Part model, mm, in its own coordinate system. A direction names the side the tool comes from. Give positions to 0.01 mm unless a question says otherwise; leave off trailing zeros. Write each loop counter-clockwise with the first axis right and the second up, starting at its lowest first coordinate (ties: lowest second). Pieces come first, ordered by that corner, then holes. Notation, with made-up numbers: M 20.5,23.5 L 71.5,23.5 A20 cw 71.5,34.5 Z; hole C -31,2 d2. An arc over 180 degrees is marked long. Write item = value, one per line. Start each with the question number.
from build123d import *

# Parameters (mm, degrees)
SKETCH_2_R          = 3
SKETCH_2_R_2        = 0.75
CUT_EXTRUDE_1_DEPTH = 10
EXTRUDE_START       = -3.5
SKETCH_3_R          = 3
SKETCH_3_R_2        = 1.5
EXTRUDE_1_DEPTH     = 2.9


with BuildPart() as part:
    # 草图1 → 旋转1 (revolve)
    with BuildSketch(Plane.XY, mode=Mode.PRIVATE) as revolve_1_sk:
        Polygon((0, -0.6), (-3.55, -0.6), (-4.836704152, 0), (-10.35, 0), (-10.35, 2.6), (-4.3, 2.6), (-4.3, 5.8), (0, 5.8), align=None)
    revolve(revolve_1_sk.sketch.rotate(Axis((0, 0, 0), (0, 1, 0)), 270), axis=Axis((0, 0, 0), (0, 1, 0)))

    # 草图2 → 切除-拉伸1 (cut)
    with BuildSketch(Plane(origin=(0, 5.8, 0), x_dir=(1, 0, 0), z_dir=(0, 1, 0))):
        with Locations(Location((0, 0, 0), (0, 0, 270))):
            Circle(SKETCH_2_R)
        with Locations(Location((0, 7.25, 0), (0, 0, 270))):
            Circle(SKETCH_2_R_2)
        with Locations(Location((7.25, 0, 0), (0, 0, 270))):
            Circle(SKETCH_2_R_2)
        with Locations(Location((0, -7.25, 0), (0, 0, 270))):
            Circle(SKETCH_2_R_2)
        with Locations(Location((-7.25, 0, 0), (0, 0, 270))):
            Circle(SKETCH_2_R_2)
    extrude(amount=-CUT_EXTRUDE_1_DEPTH, mode=Mode.SUBTRACT)

    # 草图3 → 凸台-拉伸1 (add)
    with BuildSketch(Plane(origin=(0, 5.8, 0), x_dir=(1, 0, 0), z_dir=(0, 1, 0)).offset(EXTRUDE_START)):
        with Locations(Location((0, 0, 0), (0, 0, 270))):
            Circle(SKETCH_3_R)
        with Locations(Location((0, 0, 0), (0, 0, 270))):
            Circle(SKETCH_3_R_2, mode=Mode.SUBTRACT)
    extrude(amount=-EXTRUDE_1_DEPTH)


solid = part.part
Q1. Slice it at B-B (z = 0). Give the cut face in (x, y), and give its area (3 significant figures).
Q2. Slice it at C-C (y = 0.5). Give the cut face in (x, z), and give its area (3 significant figures).
Q3. Slice it at D-D (z = 7.25). Give the cut face in (x, y).
Q4. Drop flat-ended pins along their axis: P1, Ø3, axis at x = 4, y = 3.5, coming from the -Z side; P2, Ø4, axis at x = -8, z = -8, coming from the -Y side; P3, Ø2, axis at x = 4, y = 4.5, coming from the -Z side. Give the stop position or say it passes through.
Q5. Slice it at A-A (x = 0). Give the cut face in (y, z), and give its area (3 significant figures).
Q6. Tool access for faces 1 (the face through (-1.3, 2.3, 1.3)), 2 (the face through (4.5, 0, 2.2)), 3 (the face through (-2, -0.6, 0)): list every direction of +Z, -Z, +X, -X, +Y, -Y with a clear straight run to the whole face (end or side of a thin tool).
Q7. Probe line 1 along X through (y, z) = (1.1, 0); line 2 along Y through (x, z) = (-7.25, 4.25); line 3 along X through (y, z) = (1.05, -7.25). List the from-to ranges inside material, lowest first.
Working result:
q1.outline = M -10.35,0 L -8,0 L -8,2.6 L -10.35,2.6 Z; M -6.5,0 L -4.84,0 L -3.55,-0.6 L -1.5,-0.6 L -1.5,2.3 L -3,2.3 L -3,5.8 L -4.3,5.8 L -4.3,2.6 L -6.5,2.6 Z; M 1.5,-0.6 L 3.55,-0.6 L 4.84,0 L 6.5,0 L 6.5,2.6 L 4.3,2.6 L 4.3,5.8 L 3,5.8 L 3,2.3 L 1.5,2.3 Z; M 8,0 L 10.35,0 L 10.35,2.6 L 8,2.6 Z
q1.area = 48.9 mm2
q2.outline = C 0,0 d20.7; hole C -7.25,0 d1.5; hole C 0,0 d3; hole C 0,-7.25 d1.5; hole C 0,7.25 d1.5; hole C 7.25,0 d1.5
q2.area = 322 mm2
q3.outline = M -7.39,0 L -0.75,0 L -0.75,2.6 L -7.39,2.6 Z; M 0.75,0 L 7.39,0 L 7.39,2.6 L 0.75,2.6 Z
q4.P1 = -9.96
q4.P2 = 0
q4.P3 = -3.08
q5.outline = M -0.6,-3.55 L 0,-4.84 L 0,-6.5 L 2.6,-6.5 L 2.6,-4.3 L 5.8,-4.3 L 5.8,-3 L 2.3,-3 L 2.3,-1.5 L -0.6,-1.5 Z; M -0.6,1.5 L 2.3,1.5 L 2.3,3 L 5.8,3 L 5.8,4.3 L 2.6,4.3 L 2.6,6.5 L 0,6.5 L 0,4.84 L -0.6,3.55 Z; M 0,-10.35 L 2.6,-10.35 L 2.6,-8 L 0,-8 Z; M 0,8 L 2.6,8 L 2.6,10.35 L 0,10.35 Z
q5.area = 48.9 mm2
q6.face_1 = +Y
q6.face_2 = -Y
q6.face_3 = +Z, -Z, +X, -X, -Y
q7.line_1 = -10.35 to -8, -6.5 to -1.5, 1.5 to 6.5, 8 to 10.35
q7.line_2 = 0 to 2.6
q7.line_3 = -7.39 to -0.75, 0.75 to 7.39
